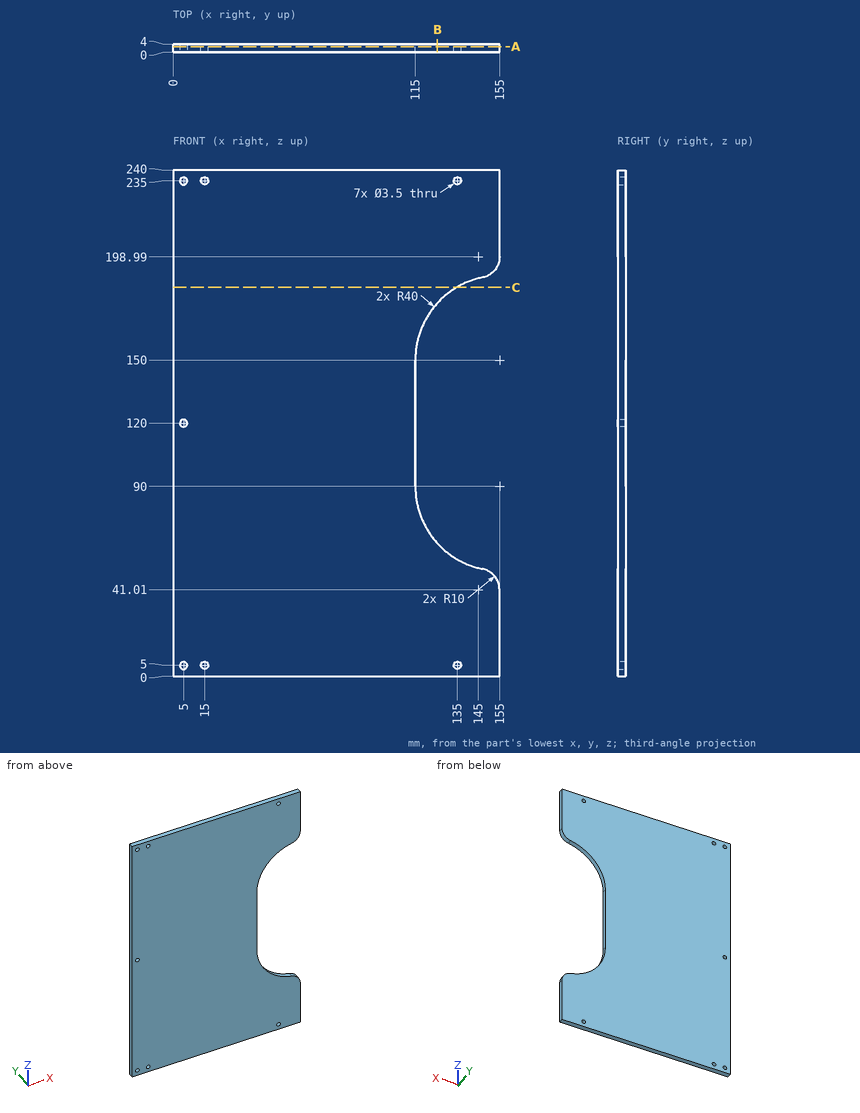
For this review, use the dimensioned drawing (mm, ordinates from the lowest corner) and the shaded views. Round coordinates to 2 decimals unless told otherwise and drop trailing zeros. Order: outer loops, then holes, each group sorted by start corner. A loop starts at its lowest first (then second) coordinate and runs counter-clockwise, first axis right, second up.
1) Consider section C-C (z = 184.5). State the section outline as (x, y) points.
The answers:
outline: (0, 0) - (134.76, 0) - (134.76, 4) - (0, 4) - close
2) Consider section A-A (y = 2.75). State the section outline as (x, z) points, plus the area to 3 significant figures.
The answers:
outline: (0, 0) - (155, 0) - (155, 41.01) arc R10 ccw to (147, 50.81) arc R40 cw to (115, 90) - (115, 150) arc R40 cw to (147, 189.19) arc R10 ccw to (155, 198.99) - (155, 240) - (0, 240) - close; hole circle Ø3.5 at (5, 5); hole circle Ø3.5 at (5, 120); hole circle Ø3.5 at (5, 235); hole circle Ø3.5 at (15, 5); hole circle Ø3.5 at (15, 235); hole circle Ø3.5 at (135, 5); hole circle Ø3.5 at (135, 235)
area: 32,200 mm2
3) Consider section B-B (x = 125.5). State the section outline as (y, z) points.
The answers:
outline: (0, 0) - (4, 0) - (4, 62.99) - (0, 62.99) - close; (0, 177.01) - (4, 177.01) - (4, 240) - (0, 240) - close
4) Clearance check with flat-ended pins moving along their axes: pin 1 Ø3 at (x, z) = (15, 5) entering from -Y; pin 2 Ø4.5 at (x, z) = (5, 120) entering from +Y. State where each tip first meets the part, or that it passes through.
The answers:
pin 1: passes through
pin 2: stops at y = 4
5) For L1, parallel to Z at x = 15, y = 1.6; L2, parallel to Z at x = 5, y = 1; L3, parallel to X at y = 2, z = 235, list the stretches that pass through material, from the lowest coordinate up.
The answers:
L1: z = 0 to 3.25, 6.75 to 233.25, 236.75 to 240
L2: z = 0 to 3.25, 6.75 to 118.25, 121.75 to 233.25, 236.75 to 240
L3: x = 0 to 3.25, 6.75 to 13.25, 16.75 to 133.25, 136.75 to 155
